Part model, mm, in its own coordinate system. A direction names the side the tool comes from. Round coordinates to 2 decimals unless told otherwise and drop trailing zeros. Loops run counter-clockwise (first coordinate to the right, second up) from the corner with the lowest first, then second, coordinate; pieces in that order, holes last. Notation, with made-up numbers: (52, -19) - (102, -19) arc R9 ccw to (102, -4) - close; hole circle Ø5 at (22.5, -22). An arc over 180 degrees is marked (long way). Put each result on its own line as item: value.
from build123d import *

# Parameters (mm, degrees)
F0_W     = 139.7
F0_H     = 25.4
F1_DEPTH = 12.7
F2_R     = 12.7
F3_DEPTH = 12.701


# Not quite as in the source:
# - a feature names something its author has since deleted; it is built from what else it names


with BuildPart() as f1:
    # F0 (on Top) → F1 (new body)
    with BuildSketch(Plane.XY):
        Polygon((0, 127), (0, 0), (279.4, 0), (279.4, 127), (139.7, 127), align=None)
        with Locations((209.55, 139.7)):
            Rectangle(F0_W, F0_H)
    extrude(amount=F1_DEPTH)

    # F2 (on face) → F3 (cut, through all)
    with BuildSketch(Plane.XY.offset(12.7)):
        with Locations((228.6, 120.65)):
            Circle(F2_R)
    extrude(amount=-F3_DEPTH, mode=Mode.SUBTRACT)


solid = f1.part
1. Two-plate mould, pull along X, no slides. Class faces 1 (the cylindrical face through (215.912, 121.208, 6.439)), 2 (the flat face through (138, 0, 6)), 3 (the flat face through (139.7, 140, 6)), 4 (the flat face through (279.4, 75, 6)): pulls with the +X half, pulls with the -X half, needs draft (parallel to the pull), parting line crosses it, or undercut.
A:
face 1: undercut
face 2: needs draft
face 3: pulls with the -X half
face 4: pulls with the +X half
2. Band-saw the part on B-B (z = 3.25). List the corners of the cut face in (x, y), plus the area to 3 significant figures.
A:
outline: (0, 0) - (279.4, 0) - (279.4, 152.4) - (139.7, 152.4) - (139.7, 127) - (0, 127) - close; hole circle Ø25.4 at (228.6, 120.65)
area: 38,500 mm²
3. Band-saw the part on D-D (x = 66.5). List the corners of the cut face in (y, z), plus the area to 3 significant figures.
A:
outline: (0, 0) - (127, 0) - (127, 12.7) - (0, 12.7) - close
area: 1,610 mm²
4. Band-saw the part on A-A (x = 228.6). List the corners of the cut face in (y, z).
A:
outline: (0, 0) - (107.95, 0) - (107.95, 12.7) - (0, 12.7) - close; (133.35, 0) - (152.4, 0) - (152.4, 12.7) - (133.35, 12.7) - close
5. Band-saw the part on C-C (y = 120.65). List the corners of the cut face in (x, z), plus the area to 3 significant figures.
A:
outline: (0, 0) - (215.9, 0) - (215.9, 12.7) - (0, 12.7) - close; (241.3, 0) - (279.4, 0) - (279.4, 12.7) - (241.3, 12.7) - close
area: 3,230 mm²
6. Pin check, flat tips, straight feed: P1, Ø1, axis at x = 118, z = 5.5, coming from the +Y side; P2, Ø4, axis at y = 136.5, z = 6, coming from the -X side. Stop position of each tip, or through.
A:
P1: stops at y = 127
P2: stops at x = 139.7
7. Probe line 1 along Y through (x, z) = (228.6, 4); line 2 along Y through (x, z) = (44.5, 5.5); line 3 along X through (y, z) = (119, 3.5). List the from-to ranges inside material, lowest first. Write a range as [from, to].
A:
line 1: y = [0, 107.95], [133.35, 152.4]
line 2: y = [0, 127]
line 3: x = [0, 216.01], [241.19, 279.4]
8. Tool access for faces 5 (the flat face through (138, 60, 12.7)), 6 (the flat face through (71, 127, 6)): list every direction of +Z, -Z, +X, -X, +Y, -Y with a clear straight run to the whole face (end or side of a thin tool).
A:
face 5: +Z, +X, -X, +Y, -Y
face 6: +Z, -Z, -X, +Y
